The listing builds one solid part. Answer for the finished solid, in the listing's coordinates (mm). A direction names the side the tool comes from. Coordinates: 2 decimals unless noted, no trailing zeros. Order: outer loops, then holes, each group sorted by start corner. A loop starts at its lowest first (then second) coordinate and runs counter-clockwise, first axis right, second up. Notation, with made-up numbers: (-14, 89.5) -> (23, 89.5) arc R15 ccw to (23, 94.5) -> close; hole circle Ø9 at (36.5, 43.25). An arc over 180 degrees is marked (long way). One line per question, with ' | ' between items.
from build123d import *

# Parameters (mm, degrees)
SKETCH1_R           = 19.1135
SKETCH1_R_2         = 3.302
BOSS_EXTRUDE1_DEPTH = 25.4
SKETCH1_4_R         = 19.1135
BOSS_EXTRUDE2_DEPTH = 12.7


with BuildPart() as part:
    # Sketch1 → Boss-Extrude1 (new body)
    with BuildSketch(Plane.XY):
        with BuildLine():
            Line((6.4262, -41.275), (6.4262, -50.391903651))
            ThreePointArc((6.4262, -50.391903651), (0, 50.8), (-6.4262, -50.391903651))
            Line((-6.4262, -50.391903651), (-6.4262, -41.275))
            Line((-6.4262, -41.275), (6.4262, -41.275))
        make_face()
        Circle(SKETCH1_R, mode=Mode.SUBTRACT)
        with Locations((-25.4, 0)):
            Circle(SKETCH1_R_2, mode=Mode.SUBTRACT)
        with Locations((0, -25.4)):
            Circle(SKETCH1_R_2, mode=Mode.SUBTRACT)
        with Locations((25.4, 0)):
            Circle(SKETCH1_R_2, mode=Mode.SUBTRACT)
        with Locations((0, 25.4)):
            Circle(SKETCH1_R_2, mode=Mode.SUBTRACT)
        Circle(SKETCH1_R)
    extrude(amount=-BOSS_EXTRUDE1_DEPTH)

    # Sketch1_4 → Boss-Extrude2 (add)
    with BuildSketch(Plane.XY):
        Circle(SKETCH1_4_R)
    extrude(amount=BOSS_EXTRUDE2_DEPTH)


solid = part.part
Item 1: Determine the mould class of faces 1 (the face through (2.143, 50.755, -12.522)), 2 (the face through (6.426, -46, -13)), 3 (the face through (0, 0, 12.7)) for opening direction X: pulls with the +X half, pulls with the -X half, needs draft (parallel to the pull), parting line crosses it, or undercut.
Computed values:
face 1: parting line crosses it | face 2: undercut | face 3: needs draft
Item 2: For faces 4 (the face through (-14.087, 12.918, 6.261)), 5 (the face through (-0.43, 28.674, -12.522)), 6 (the face through (0, -41.275, -13)), determine the directions among +Z, -Z, +X, -X, +Y, -Y from which every point of the face is accessible in a straight line to the end or side of a thin tool.
Computed values:
face 4: +Z | face 5: +Z, -Z | face 6: +Z, -Z, -Y
Item 3: Section D-D, the plane y = 25.4 is taken. Give the vertices of the cut face in (x, z).
Computed values:
outline: (-43.99, -25.4) -> (-3.3, -25.4) -> (-3.3, 0) -> (-43.99, 0) -> close; (3.3, -25.4) -> (43.99, -25.4) -> (43.99, 0) -> (3.3, 0) -> close
Item 4: Each of these flat-tipped pins is pushed along its axis until it touches: pin 1 Ø4.5 at (y, z) = (-44.5, -12.5) entering from -X; pin 2 Ø3 at (x, z) = (24.5, -18) entering from -Y; pin 3 Ø7.5 at (x, y) = (0, -25.4) entering from +Z; pin 4 Ø4 at (x, y) = (0, 25.4) entering from +Z. Where does it stop, or does it pass through?
Computed values:
pin 1: stops at x = -28.21 | pin 2: stops at y = -45.3 | pin 3: stops at z = 0 | pin 4: passes through
Item 5: Section B-B, the plane z = -16 is taken. Give the vertices of the cut face in (x, y) (3 decimals), plus the area to 3 significant figures.
Computed values:
outline: (-6.426, -50.392) -> (-6.426, -41.275) -> (6.426, -41.275) -> (6.426, -50.392) arc R50.8 ccw (long way) to start; hole circle Ø6.604 at (-25.4, 0); hole circle Ø6.604 at (0, -25.4); hole circle Ø6.604 at (0, 25.4); hole circle Ø6.604 at (25.4, 0) | area: 7,850 mm^2
Item 6: Section A-A, the plane x = 0 is taken. Give the vertices of the cut face in (y, z) (1 decimal).
Computed values:
outline: (-41.3, -25.4) -> (-28.7, -25.4) -> (-28.7, 0) -> (-41.3, 0) -> close; (-22.1, -25.4) -> (22.1, -25.4) -> (22.1, 0) -> (19.1, 0) -> (19.1, 12.7) -> (-19.1, 12.7) -> (-19.1, 0) -> (-22.1, 0) -> close; (28.7, -25.4) -> (50.8, -25.4) -> (50.8, 0) -> (28.7, 0) -> close
Item 7: Find the intervals of material crossed by L1, parallel to Y at x = 0, z = -11.75 (3 decimals); L2, parallel to X at y = -2, z = -12; L3, parallel to Z at x = -27, y = -29.5, in increasing order.
Computed values:
L1: y = -41.275 to -28.702, -22.098 to 22.098, 28.702 to 50.8 | L2: x = -50.76 to -28.03, -22.77 to 22.77, 28.03 to 50.76 | L3: z = -25.4 to 0
Item 8: Section C-C, the plane x = 25 is taken. Give the vertices of the cut face in (y, z), plus the area to 3 significant figures.
Computed values:
outline: (-44.22, -25.4) -> (-3.28, -25.4) -> (-3.28, 0) -> (-44.22, 0) -> close; (3.28, -25.4) -> (44.22, -25.4) -> (44.22, 0) -> (3.28, 0) -> close | area: 2,080 mm^2
